Could you check a few things on this model? Use its own coordinates, in mm. Round coordinates to 2 decimals unless told otherwise and drop trailing zeros. Write each loop counter-clockwise with the first axis right and the second up, starting at its lowest first coordinate (ties: lowest second). Pieces come first, ordered by that corner, then holes.
```python
from build123d import *

# Parameters (mm, degrees)
CROQUIS1_R              = 2.5
SALIENTE_EXTRUIR1_DEPTH = 326
SKETCH2_W               = 139.582587955
SKETCH2_H               = 242.432915921
CUT_EXTRUDE1_DEPTH      = 47
CUT_EXTRUDE1_DEPTH_BACK = 30


with BuildPart() as part:
    # Croquis1 → Saliente-Extruir1 (new body)
    with BuildSketch(Plane.XY):
        with BuildLine():
            Line((-4.6, 10), (-3.1, 8.5))
            Line((-3.1, 8.5), (-3.1, 8.2))
            Line((-3.1, 8.2), (-5.5, 8.2))
            Line((-5.5, 8.2), (-5.5, 6.560660172))
            Line((-5.5, 6.560660172), (-2.84, 3.900660172))
            Line((-2.84, 3.900660172), (0, 3.900660172))
            Line((0, 3.900660172), (2.84, 3.900660172))
            Line((2.84, 3.900660172), (5.5, 6.560660172))
            Line((5.5, 6.560660172), (5.5, 8.2))
            Line((5.5, 8.2), (3.1, 8.2))
            Line((3.1, 8.2), (3.1, 8.5))
            Line((3.1, 8.5), (4.6, 10))
            Line((4.6, 10), (9.25, 10))
            ThreePointArc((9.25, 10), (9.780330086, 9.780330086), (10, 9.25))
            Line((10, 9.25), (10, 4.6))
            Line((10, 4.6), (8.5, 3.1))
            Line((8.5, 3.1), (8.2, 3.1))
            Line((8.2, 3.1), (8.2, 5.5))
            Line((8.2, 5.5), (6.560660172, 5.5))
            Line((6.560660172, 5.5), (3.900660172, 2.84))
            Line((3.900660172, 2.84), (3.900660172, 0))
            Line((3.900660172, 0), (3.900660172, -2.84))
            Line((3.900660172, -2.84), (6.560660172, -5.5))
            Line((6.560660172, -5.5), (8.2, -5.5))
            Line((8.2, -5.5), (8.2, -3.1))
            Line((8.2, -3.1), (8.5, -3.1))
            Line((8.5, -3.1), (10, -4.6))
            Line((10, -4.6), (10, -9.25))
            ThreePointArc((10, -9.25), (9.780330086, -9.780330086), (9.25, -10))
            Line((9.25, -10), (4.6, -10))
            Line((4.6, -10), (3.1, -8.5))
            Line((3.1, -8.5), (3.1, -8.2))
            Line((3.1, -8.2), (5.5, -8.2))
            Line((5.5, -8.2), (5.5, -6.560660172))
            Line((5.5, -6.560660172), (2.84, -3.900660172))
            Line((2.84, -3.900660172), (0, -3.900660172))
            Line((0, -3.900660172), (-2.84, -3.900660172))
            Line((-2.84, -3.900660172), (-5.5, -6.560660172))
            Line((-5.5, -6.560660172), (-5.5, -8.2))
            Line((-5.5, -8.2), (-3.1, -8.2))
            Line((-3.1, -8.2), (-3.1, -8.5))
            Line((-3.1, -8.5), (-4.6, -10))
            Line((-4.6, -10), (-9.25, -10))
            ThreePointArc((-9.25, -10), (-9.780330086, -9.780330086), (-10, -9.25))
            Line((-10, -9.25), (-10, -4.6))
            Line((-10, -4.6), (-8.5, -3.1))
            Line((-8.5, -3.1), (-8.2, -3.1))
            Line((-8.2, -3.1), (-8.2, -5.5))
            Line((-8.2, -5.5), (-6.560660172, -5.5))
            Line((-6.560660172, -5.5), (-3.900660172, -2.84))
            Line((-3.900660172, -2.84), (-3.900660172, 0))
            Line((-3.900660172, 0), (-3.900660172, 2.84))
            Line((-3.900660172, 2.84), (-6.560660172, 5.5))
            Line((-6.560660172, 5.5), (-8.2, 5.5))
            Line((-8.2, 5.5), (-8.2, 3.1))
            Line((-8.2, 3.1), (-8.5, 3.1))
            Line((-8.5, 3.1), (-10, 4.6))
            Line((-10, 4.6), (-10, 9.25))
            ThreePointArc((-10, 9.25), (-9.780330086, 9.780330086), (-9.25, 10))
            Line((-9.25, 10), (-4.6, 10))
        make_face()
        Circle(CROQUIS1_R, mode=Mode.SUBTRACT)
    extrude(amount=SALIENTE_EXTRUIR1_DEPTH)

    # Sketch2 → Cut-Extrude1 (cut, two sides)
    with BuildSketch(Plane(origin=(0, 0, 0), x_dir=(1, 0, 0), z_dir=(0, 1, 0))) as cut_extrude1_sk:
        with Locations((12.355396541, -401.216457961)):
            Rectangle(SKETCH2_W, SKETCH2_H)
    extrude(amount=CUT_EXTRUDE1_DEPTH, mode=Mode.SUBTRACT)
    extrude(cut_extrude1_sk.sketch, amount=-CUT_EXTRUDE1_DEPTH_BACK, mode=Mode.SUBTRACT)


solid = part.part
```
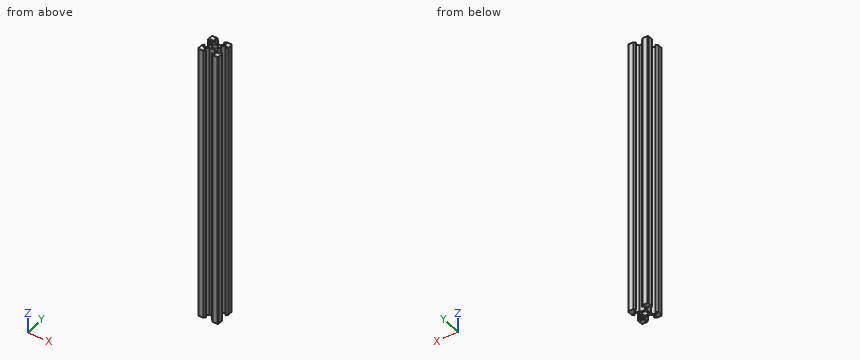
Q1. I'm going to push flat-ended pins straight in: pin 1 Ø6 at (x, z) = (1, 97) entering from +Y; pin 2 Ø6 at (y, z) = (-1, 209) entering from -X; pin 3 Ø2 at (y, z) = (2, 160) entering from -X; pin 4 Ø4.5 at (x, y) = (0, 0) entering from -Z. Where does each tip first touch, or does it pass through?
Q2. If I drill on L1, parallel to X at y = 0, z = 101.5; L2, parallel to X at y = -4.25, z = 236, over which ranges is the centre line in solid material (lowest first)?
Q3. Imagine slicing it at A-A, the plane y = 0. Write out the boundary of the cut face in (x, z), then the cut area to 3 significant figures.
Results found:
1. pin 1: stops at y = 9.4
1. pin 2: stops at x = -9.4
1. pin 3: stops at x = -4.06
1. pin 4: passes through
2. L1: x = -3.9 to -2.5, 2.5 to 3.9
2. L2: x = -9.65 to -8.2, -5.31 to -3.19, 3.19 to 5.31, 8.2 to 9.65
3. outline: (-3.9, 0) - (-2.5, 0) - (-2.5, 280) - (-3.9, 280) - close; (2.5, 0) - (3.9, 0) - (3.9, 280) - (2.5, 280) - close
3. area: 784 mm2
